Job drawing, mm, ordinate dimensions from the low corner. One solid piece. A direction names the side the tool comes from. Give positions to 0.01 mm unless a question says otherwise; leave off trailing zeros. Write each loop counter-clockwise with the first axis right and the second up, starting at its lowest first coordinate (ties: lowest second). Pieces come first, ordered by that corner, then holes. Notation, with made-up numbers: (17, 42.25) -> (55, 42.25) arc R23 cw to (55, 54.25) -> close; hole circle Ø7 at (12.5, -10.75). An arc over 180 degrees is marked (long way). Put each result on its own line as item: value. Start each with the question number.
Item 1: Flat gauge pin, fed straight in: pin 1 Ø12 at (x, y) = (34.5, 31) entering from -Z. Where does the tip first touch, or does it go through?
Item 2: Slice it at A-A, the plane x = 32.5. List the corners of the cut face in (y, z), plus the area to 3 significant figures.
Item 3: Slice it at C-C, the plane z = 45. List the corners of the cut face in (x, y), plus the area to 3 significant figures.
Item 4: Slice it at D-D, the plane x = 49. List the corners of the cut face in (y, z).
Item 5: Drill centre lines: line 1 along X through (y, z) = (32, 7); line 2 along Y through (x, z) = (32.5, 40.5); line 3 along Z through (x, y) = (36, 41.5). Where is each one in solid material? Low to high.
Item 6: Tool access for the marked faces 1 and 2: list every direction of +Z, -Z, +X, -X, +Y, -Y with a clear straight run to the whole face (end or side of a thin tool).
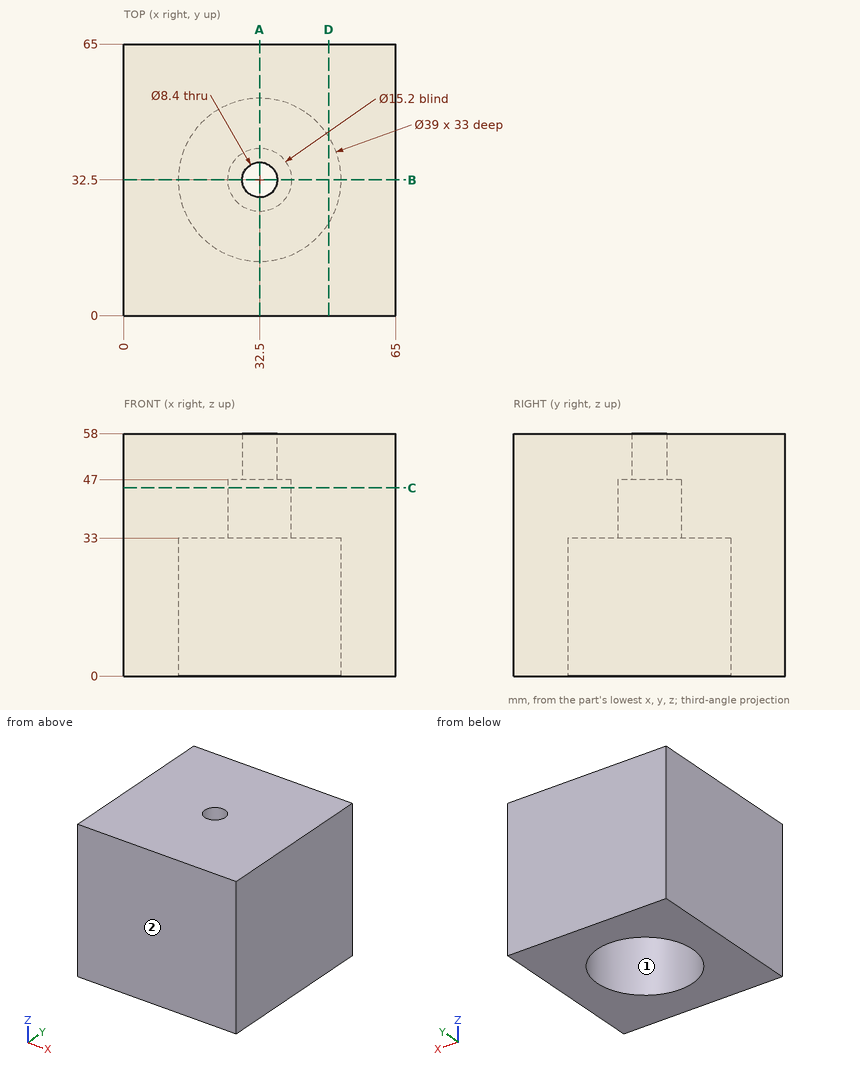
Values follow:
1. pin 1: z = 33
2. outline: (0, 0) -> (13, 0) -> (13, 33) -> (24.9, 33) -> (24.9, 47) -> (28.3, 47) -> (28.3, 58) -> (0, 58) -> close; (36.7, 47) -> (40.1, 47) -> (40.1, 33) -> (52, 33) -> (52, 0) -> (65, 0) -> (65, 58) -> (36.7, 58) -> close
2. area: 2,180 mm2
3. outline: (0, 0) -> (65, 0) -> (65, 65) -> (0, 65) -> close; hole circle Ø15.2 at (32.5, 32.5)
3. area: 4,040 mm2
4. outline: (0, 0) -> (22.11, 0) -> (22.11, 33) -> (42.89, 33) -> (42.89, 0) -> (65, 0) -> (65, 58) -> (0, 58) -> close
5. line 1: 0 to 13.01, 51.99 to 65
5. line 2: 0 to 24.9, 40.1 to 65
5. line 3: 33 to 58
6. face 1: -Z
6. face 2: +Z, -Z, +X, -X, -Y
